Verification items for the finished model (mm, model axes). Face numbers are marked on the shaded views. A direction names the side the tool comes from. Round coordinates to 2 decimals unless told otherwise and drop trailing zeros. Write each loop counter-clockwise with the first axis right and the second up, starting at its lowest first coordinate (ties: lowest second). Pieces come first, ordered by that corner, then holes. Notation, with made-up numbers: (56.25, 71.5) - (76.25, 71.5) arc R23 ccw to (76.25, 96.5) - close; hole circle Ø11 at (80, 56.5). An arc over 180 degrees is marked (long way). Answer as a JSON object with one key per item and string values. Group by question number.
1) Go/stop test with flat-tipped pins: pin 1 Ø1.5 at (x, z) = (19, 8) entering from -Y; pin 2 Ø3 at (x, z) = (21.5, 2.5) entering from -Y; pin 3 Ø1 at (x, z) = (-11, 7.5) entering from +Y; pin 4 Ø3 at (x, z) = (0.5, 6) entering from -Y. Record where each tip stops, or that it passes through.
2) Section check B-B (z = 9.5). Enter the section's corners in (x, y), then the cut area to 3 significant figures.
3) Thickness scan on line 1 (Y direction, x = -24.5, z = 7); line 2 (Z direction, x = 0, y = -0.55); line 3 (X direction, y = -9.5, z = 12). Record the ranges inside material, lowest first.
4) Mould release check, pull along Y, two halves, no side actions. Record for the marked faces 4, 5 and 6: +Y half, -Y half, draft (parallel to the pull), parting line (faces both ways), or undercut.
5) Set-up check for the marked faces 1, 2 and 3: record each of +Z, -Z, +X, -X, +Y, -Y from which the full face is reachable in a straight line by a thin tool's end or side.
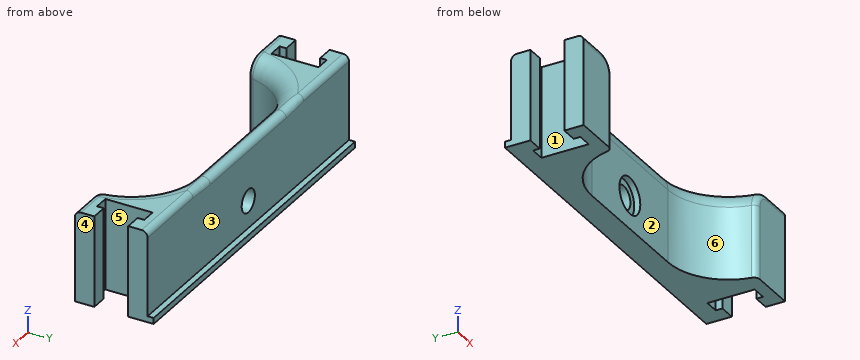
```python
from build123d import *

# Parameters (mm, degrees)
F0_W           = 58
F0_H           = 15
F2_DEPTH       = 12
F4_DEPTH       = 25
F5_W           = 41.8
F5_H           = 9
F6_DEPTH       = 25
F1_W           = 58
F1_H           = 1
F8_DEPTH       = 1
F9_D           = 3.8
F9_CBORE_D     = 6
F9_CBORE_DEPTH = 1
F10_T1_DEPTH   = 15
F11_R          = 2.99999
F12_R          = 1
F13_R          = 1


# Not quite as in the source:
# - a fillet or chamfer that OpenCascade refuses, or shapes differently, is made with other operations: its cross-section is extruded or revolved along the edge and cut away or added
# - a fillet or chamfer is up to 0.001 mm smaller than in the source, because OpenCascade refuses the exact size


with BuildPart() as f2:
    # F0 (on Front) → F2 (new body)
    with BuildSketch(Plane.XZ):
        with Locations((0, 7.5)):
            Rectangle(F0_W, F0_H)
    extrude(amount=F2_DEPTH)

    # F3 (on Top) → F4 (cut)
    with BuildSketch(Plane.XY):
        Polygon((-26.3, -3.2), (-29, -3.2), (-29, -8.8), (-26.3, -8.8), (-26.3, -9.9), (-23.9, -9.9), (-23.9, -2.1), (-26.3, -2.1), align=None)
        Polygon((29, -8.8), (29, -3.2), (26.3, -3.2), (26.3, -2.1), (23.9, -2.1), (23.9, -9.9), (26.3, -9.9), (26.3, -8.8), align=None)
    extrude(amount=F4_DEPTH, mode=Mode.SUBTRACT)

    # F5 (on Top) → F6 (cut)
    with BuildSketch(Plane.XY):
        with Locations((0, -7.5)):
            Rectangle(F5_W, F5_H)
    extrude(amount=F6_DEPTH, mode=Mode.SUBTRACT)

    # F1 (on Front) → F8 (join)
    with BuildSketch(Plane.XZ):
        with Locations((0, 0.5)):
            Rectangle(F1_W, F1_H)
    extrude(amount=-F8_DEPTH)

    # F9 (through all)
    with Locations(Plane.XZ.offset(3)):
        with Locations((0, 5.5)):
            CounterBoreHole(F9_D / 2, F9_CBORE_D / 2, F9_CBORE_DEPTH)

    # F10: fillet of radius 10 on 2 edges, made by hand

    # F10_s2 → F10_t1 (join)
    with BuildSketch(Plane.XY):
        with BuildLine():
            ThreePointArc((-20.9, -12), (-17.6583295614, -5.5838015129), (-10.9501256289, -3))
            Line((-10.9501256289, -3), (-20.9, -3))
            Line((-20.9, -3), (-20.9, -12))
        make_face()
        with BuildLine():
            ThreePointArc((10.9501256289, -3), (17.6583295614, -5.5838015129), (20.9, -12))
            Line((20.9, -12), (20.9, -3))
            Line((20.9, -3), (10.9501256289, -3))
        make_face()
    extrude(amount=F10_T1_DEPTH)

    # F11 (radius 3 in the source; OpenCascade refuses exactly that, so slightly less here)
    f11_edges = [f2.edges().sort_by_distance(p)[0] for p in [
        (0, -3, 15),
        (17.65833, -5.583802, 15),
        (-17.65833, -5.583802, 15),
    ]]
    fillet(f11_edges, radius=F11_R)

    # F12
    f12_edges = [f2.edges().sort_by_distance(p)[0] for p in [
        (-26.455798, -12, 15),
        (26.455798, -12, 15),
    ]]
    fillet(f12_edges, radius=F12_R)

    # F13
    f13_edges = [f2.edges().sort_by_distance(p)[0] for p in [
        (0, 0, 15),
    ]]
    fillet(f13_edges, radius=F13_R)


solid = f2.part
```
Returned:
{
 "1": {"pin 1": "y = -8.25", "pin 2": "y = -12", "pin 3": "y = 0", "pin 4": "y = -2"},
 "2": {"outline": "(-29, -12) - (-21.77, -12) arc R1 ccw to (-20.78, -11.18) arc R10 cw to (-10.95, -3) - (10.95, -3) arc R10 cw to (20.78, -11.18) arc R1 ccw to (21.77, -12) - (29, -12) - (29, -8.8) - (26.3, -8.8) - (26.3, -9.9) - (23.9, -9.9) - (23.9, -2.1) - (26.3, -2.1) - (26.3, -3.2) - (29, -3.2) - (29, 0) - (-29, 0) - (-29, -3.2) - (-26.3, -3.2) - (-26.3, -2.1) - (-23.9, -2.1) - (-23.9, -9.9) - (-26.3, -9.9) - (-26.3, -8.8) - (-29, -8.8) - close", "area": "294 mm2"},
 "3": {"line 1": "-12 to -9.9, -2.1 to 0", "line 2": "0 to 3.6, 7.4 to 14.63", "line 3": "-29 to -26.3, -23.9 to -20.32, 20.32 to 23.9, 26.3 to 29"},
 "4": {"face 4": "draft", "face 5": "undercut", "face 6": "-Y half"},
 "5": {"face 1": "+Z, -Z", "face 2": "+Z, -Z, -Y", "face 3": "+Z, +X, -X, +Y"}
}
